Answer from the drawing. Dimensions are ordinates in mm from the lowest x, y and z of the part. Coordinates: 2 decimals unless noted, no trailing zeros. Write each loop counter-clockwise with the first axis right and the second up, starting at its lowest first coordinate (ties: lowest second). Pieces come first, ordered by that corner, then holes.
(1) Given P1, Ø2, axis at x = 2.5, y = 2.5, coming from the +Z side, flat-ended and moving along its own axis, determine where the tip first touches the part or whether it passes through.
(2) The part is cut by section B-B on y = 2.5. Determine the outline of the cut face in (x, z), plus the area to 3 significant figures.
(3) Straight lines are drawn through the part: line 1 (Y direction, x = 131.5, z = 0.75); line 2 (X direction, y = 31.3, z = 1); line 3 (Y direction, x = 67, z = 0.6). For each, find the intervals that lie inside material, in ascending order.
(4) The part is cut by section C-C on z = 0.3. Determine the outline of the cut face in (x, y), plus the area to 3 significant figures.
(5) The part is cut by section A-A on x = 67. Determine the outline of the cut face in (y, z).
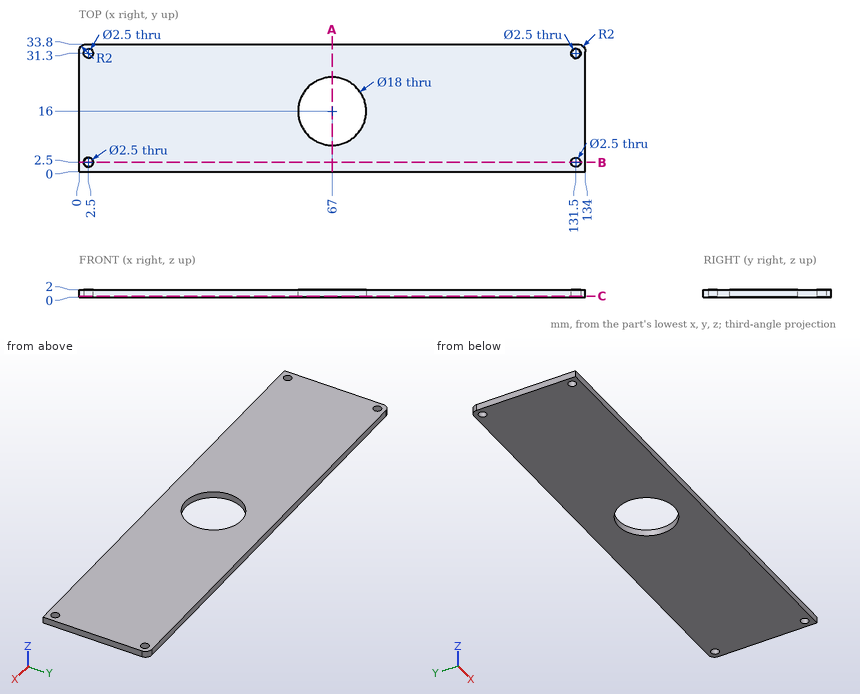
Model answer:
1. P1: passes through
2. outline: (0, 0) - (1.25, 0) - (1.25, 2) - (0, 2) - close; (3.75, 0) - (130.25, 0) - (130.25, 2) - (3.75, 2) - close; (132.75, 0) - (134, 0) - (134, 2) - (132.75, 2) - close
2. area: 258 mm2
3. line 1: y = 0 to 1.25, 3.75 to 30.05, 32.55 to 33.8
3. line 2: x = 0 to 1.25, 3.75 to 130.25, 132.75 to 134
3. line 3: y = 0 to 7, 25 to 33.8
4. outline: (0, 0) - (134, 0) - (134, 31.8) arc R2 ccw to (132, 33.8) - (2, 33.8) arc R2 ccw to (0, 31.8) - close; hole circle Ø2.5 at (2.5, 2.5); hole circle Ø2.5 at (2.5, 31.3); hole circle Ø18 at (67, 16); hole circle Ø2.5 at (131.5, 2.5); hole circle Ø2.5 at (131.5, 31.3)
4. area: 4,250 mm2
5. outline: (0, 0) - (7, 0) - (7, 2) - (0, 2) - close; (25, 0) - (33.8, 0) - (33.8, 2) - (25, 2) - close
